```python
from build123d import *

# Parameters (mm, degrees)
SKETCH1_W           = 23.85
SKETCH1_H           = 7.85
BOSS_EXTRUDE1_DEPTH = 3.15
SHELL1_T            = -1.5
SKETCH2_R           = 2.45
SKETCH2_R_2         = 1.55
BOSS_EXTRUDE2_DEPTH = 1.8


with BuildPart() as part:
    # Sketch1 → Boss-Extrude1 (new body)
    with BuildSketch(Plane(origin=(0, 0, 0), x_dir=(1, 0, 0), z_dir=(0, 1, 0))):
        Rectangle(SKETCH1_W, SKETCH1_H)
    extrude(amount=-BOSS_EXTRUDE1_DEPTH)

    # Shell1
    shell1_openings = [part.faces().sort_by_distance(p)[0] for p in [
        (0, -3.15, 0),
    ]]
    offset(amount=SHELL1_T, openings=shell1_openings, kind=Kind.INTERSECTION)

    # Sketch2 → Boss-Extrude2 (add)
    # profile 1 of 2: a face of its own
    with BuildSketch(Plane(origin=(0, 0, 0), x_dir=(1, 0, 0), z_dir=(0, 1, 0))):
        with Locations(Location((-3.975, 0, 0), (0, 0, 270))):
            Circle(SKETCH2_R)
        with Locations(Location((-3.975, 0, 0), (0, 0, 270))):
            Circle(SKETCH2_R_2, mode=Mode.SUBTRACT)
    # profile 2 of 2: a face of its own
    with BuildSketch(Plane(origin=(0, 0, 0), x_dir=(1, 0, 0), z_dir=(0, 1, 0))):
        with Locations(Location((3.975, 0, 0), (0, 0, 90))):
            Circle(SKETCH2_R)
        with Locations(Location((3.975, 0, 0), (0, 0, 90))):
            Circle(SKETCH2_R_2, mode=Mode.SUBTRACT)
    extrude(amount=BOSS_EXTRUDE2_DEPTH)


solid = part.part
```
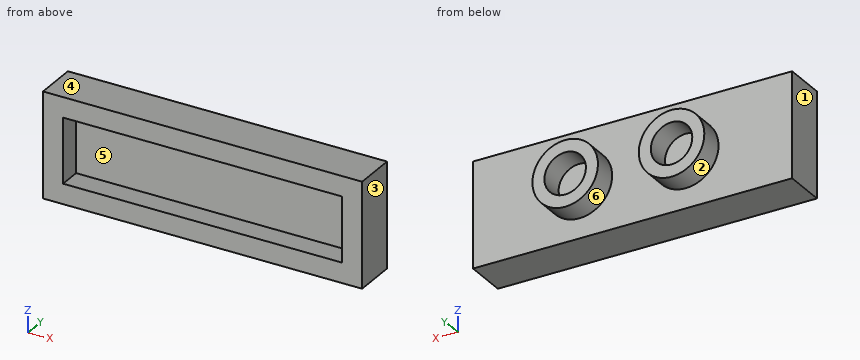
The listing builds one solid part. Answer for the finished solid, in the listing's coordinates (mm). Face numbers are marked on the shaded views. A direction names the side the tool comes from. Round coordinates to 2 decimals unless told otherwise and drop trailing zeros. Write each loop counter-clockwise with the first axis right and the second up, starting at its lowest first coordinate (ties: lowest second). Pieces come first, ordered by that corner, then holes. Notation, with made-up numbers: (19, -30.5) -> (26, -30.5) arc R12 ccw to (26, -19.5) -> close; hole circle Ø7 at (42.5, 34). An arc over 180 degrees is marked (long way). Write item = value, one per line.
1) Section D-D on y = 0.5 is taken. Write down the section's boundary in (x, z) (3 decimals), plus the area to 3 significant figures.
Check values:
outline = circle Ø4.9 at (-3.975, 0); circle Ø4.9 at (3.975, 0); hole circle Ø3.1 at (-3.975, 0); hole circle Ø3.1 at (3.975, 0)
area = 22.6 mm²
2) Which of the six approach directions +Z, -Z, +X, -X, +Y, -Y give full straight-line access (tool end or side, diameter ignored) to the marked faces 1 and 2?
Check values:
face_1 = +Z, -Z, -X, +Y, -Y
face_2 = +Y
3) Given pin 1 (0.9 mm diameter, centred on x = -4.5, z = 0, fed in from +Y); pin 2 (1.9 mm diameter, centred on x = -3.975, z = 0, fed in from -Y), each flat-ended and moving along its own axis, determine where each tip first touches the part or whether it passes through.
Check values:
pin_1 = 0
pin_2 = -1.5
4) Section C-C on z = 0 is taken. Write down the section's boundary in (x, y) (3 decimals), plus the area to 3 significant figures.
Check values:
outline = (-11.925, -3.15) -> (-10.425, -3.15) -> (-10.425, -1.5) -> (10.425, -1.5) -> (10.425, -3.15) -> (11.925, -3.15) -> (11.925, 0) -> (6.425, 0) -> (6.425, 1.8) -> (5.525, 1.8) -> (5.525, 0) -> (2.425, 0) -> (2.425, 1.8) -> (1.525, 1.8) -> (1.525, 0) -> (-1.525, 0) -> (-1.525, 1.8) -> (-2.425, 1.8) -> (-2.425, 0) -> (-5.525, 0) -> (-5.525, 1.8) -> (-6.425, 1.8) -> (-6.425, 0) -> (-11.925, 0) -> close
area = 47.2 mm²
5) Section B-B on y = -1.95 is taken. Write down the section's boundary in (x, z) (3 decimals).
Check values:
outline = (-11.925, -3.925) -> (11.925, -3.925) -> (11.925, 3.925) -> (-11.925, 3.925) -> close; hole (-10.425, -2.425) -> (10.425, -2.425) -> (10.425, 2.425) -> (-10.425, 2.425) -> close
6) For a pull along Z with two mould halves and no side action, classify the marked faces 3, 4, 5 and 6 as released by +Z, released by -Z, zero draft, split by the parting line, or undercut.
Check values:
face_3 = zero draft
face_4 = released by +Z
face_5 = undercut
face_6 = split by the parting line
7) Straight lines are drawn through the part: line 1 along X through (y, z) = (1, 0) (3 decimals); line 2 along Z through (x, y) = (8.5, -1.6) (3 decimals); line 3 along X through (y, z) = (-1.9, -0.75) (3 decimals). For each, find the intervals that lie inside material, in ascending order. Write a range as [from, to].
Check values:
line_1 = [-6.425, -5.525], [-2.425, -1.525], [1.525, 2.425], [5.525, 6.425]
line_2 = [-3.925, -2.425], [2.425, 3.925]
line_3 = [-11.925, -10.425], [10.425, 11.925]
8) Section A-A on x = 1 is taken. Write down the section's boundary in (y, z) (3 decimals), plus the area to 3 significant figures.
Check values:
outline = (-3.15, -3.925) -> (0, -3.925) -> (0, 3.925) -> (-3.15, 3.925) -> (-3.15, 2.425) -> (-1.5, 2.425) -> (-1.5, -2.425) -> (-3.15, -2.425) -> close
area = 16.7 mm²
